Autodesk Inventor part; units mm, degrees
ref_plane "YZ Plane" through (0, 0, 0) normal (1, 0, 0) x (0, 1, 0)
ref_plane "XZ Plane" through (0, 0, 0) normal (0, 1, 0) x (-1, 0, 0)
ref_plane "XY Plane" through (0, 0, 0) normal (0, 0, 1) x (1, 0, 0)
sketch "スケッチ1" plane through (0, 0, 0) normal (1, 0, 0) x (0, 1, 0)
  line L0 (-41, 550) -> (10, 550)
  line L1 (10, 550) -> (10, -10)
  line L2 (10, -10) -> (-41, -10)
  line L3 (-41, -10) -> (-41, 550)
  line L4 (-41, 550) -> (10, -10) construction
  line L5 (10, 550) -> (-41, -10) construction
  point P0 (0, 0)
  dimension "d0" = 51
  dimension "d1" = 560
  dimension "d42" = 10
  dimension "d43" = 10
extrude "プレート1" add sketch "スケッチ1" along normal mid plane 1
sketch "スケッチ3" plane through (0.5, 0, 0) normal (1, 0, 0) x (0, 0, -1)
  circle A0 centre (0, 0) radius 6
  line L0 (10, 10) -> (10, -41)
  line L1 (-550, 10) -> (10, 10)
  point P0 (0, 0)
  point P1 (0, 6)
  point P2 (-6, 0)
  point P3 (0, -6)
  point P4 (6, 0)
  dimension "d13" = 12
  dimension "d14" = 10
  dimension "d15" = 10
  dimension "d18" = 360
  dimension "d44" = 0
hole "穴2" at (0.5, 6, 0) at (0.5, 0, 6) at (0.5, -6, 0) at (0.5, 0, -6) direction (-1, 0, 0) diameter 3.2 end through all
sketch "スケッチ4" plane through (0.5, 0, 0) normal (1, 0, 0) x (0, 0, -1)
  circle A0 centre (0, 0) radius 3.05
  point P0 (0, 0)
  dimension "d27" = 6.1
extrude "押し出し1" cut sketch "スケッチ4" against normal blind 10
sketch "スケッチ5" plane through (0.5, 0, 0) normal (1, 0, 0) x (0, 0, -1)
  line L0 (10, -41) -> (-33.5, -41)
  line L1 (-33.5, -41) -> (-33.5, -10)
  line L2 (-33.5, -10) -> (10, -10)
  line L3 (10, -10) -> (10, -41)
  line L4 (-550, 10) -> (-53.5, 10)
  line L5 (-53.5, 10) -> (-53.5, -12)
  line L6 (-53.5, -12) -> (-550, -12)
  line L7 (-550, -12) -> (-550, 10)
  line L8 (10, -41) -> (-550, -41)
  circle A0 centre (0, 0) radius 3.05
  circle A1 centre (0, 0) radius 3.05
  line L9 (0, 3.05) -> (10, 3.05)
  line L10 (0, -3.05) -> (10, -3.05)
  line L11 (10, 10) -> (10, -41)
  circle A2 centre (0, 0) radius 10
  circle A3 centre (0, 6) radius 1.6
  circle A4 centre (0, -6) radius 1.6
  line L12 (-550, 10) -> (10, 10)
  line L13 (2.95, 10) -> (2.95, -10)
  point P0 (0, 0)
  point P1 (2.95, -3.05)
  point P2 (2.95, 3.05)
  point P3 (2.95, 0.7746)
  point P4 (2.95, -0.7746)
  point P5 (9.5235, -3.05)
  point P6 (0, -10)
  point P7 (0, 10)
  point P8 (9.5235, 3.05)
  point P9 (10, 0)
  point P10 (2.95, -9.555)
  point P11 (2.95, 9.555)
  dimension "d35" = 29
  dimension "d36" = 20
  dimension "d40" = 33.5
  dimension "d41" = 10
  dimension "d45" = 2.95
extrude "押し出し2" cut sketch "スケッチ5" against normal blind 10 contours L0 L1 L2 L3 | L2 L13 A2 L10 L11 | L2 A2 L13 | L10 A2 L11 | L13 L10 A2 | L10 L13 A0 L9 A2 | A2 L9 L11 | L12 L13 A2 | L10 A0 L13 | L9 A2 L13 L12 L11 | L9 L13 A2 | L13 A0 L9 picked at (5.1412, -2.2915)
fillet "コーナーR4" radius 1 4 edges at (0, -3.05, -2.95) (0, 3.05, -2.95) (0, 9.555, -2.95) (0, -9.555, -2.95)
sketch "スケッチ6" plane through (0.5, 0, 0) normal (1, 0, 0) x (0, 0, -1)
  line L0 (-33.5, -41) -> (-550, -41)
  line L1 (-33.5, -41) -> (-33.5, -10)
  line L2 (-33.5, -25) -> (-124.2405, -41)
  point P0 (0, 0)
  point P1 (-545, -41)
  point P2 (-33.5, -15)
  dimension "d51" = 10
  dimension "d52" = 16
extrude "押し出し3" cut sketch "スケッチ6" against normal blind 10
fillet "コーナーR5" radius 5 2 edges at (0, -25, 33.5) (0, -41, 124.2405)
fillet "コーナーR6" radius 5 2 edges at (0, -10, 33.5) (0, 10, 550)
equation "\"d25\" = Thickness"
equation "\"d2\" = Thickness"
equation "\"BendRadius\" = Thickness"
equation "\"BendReliefWidth\" = Thickness"
equation "\"BendReliefDepth\" = 0.5 * Thickness"
equation "\"CornerReliefSize\" = 4 * Thickness"
equation "\"MinimumRemnant\" = 2 * Thickness"
equation "\"TransitionRadius\" = BendRadius"
equation "\"JacobiRadiusSize\" = BendRadius"
equation "\"GapSize\" = Thickness"
properties part number "s_carbon_plate5" material "CFRP"
Source: CAD feature listing. Evaluate the final solid. Frame: model axes, mm. Coordinates: 2 decimals unless noted, no trailing zeros. Write each loop counter-clockwise with the first axis right and the second up, starting at its lowest first coordinate (ties: lowest second). Pieces come first, ordered by that corner, then holes. Notation, with made-up numbers: (77.25, -21.75) - (98.25, -21.75) arc R9 cw to (98.25, -17.75) - close; hole circle Ø4 at (13.5, 83.5). An arc over 180 degrees is marked (long way). Answer as a JSON object with one key per item and string values.
Q1. Section query B-B, the plane y = -31.5. Output: boundary loops of the cut face in (x, z).
Ans:
{"outline": "(-0.5, 70.36) - (0.5, 70.36) - (0.5, 550) - (-0.5, 550) - close"}
Q2. First-contact query: pin 1 Ø0.5 at (x, z) = (0, -1.5) entering from +Y. Flat tip, straight axial feed; report the tip coordinate or a pass-through.
Ans:
{"pin 1": "stops at y = 9.92"}
Q3. Section query A-A, the plane x = -0.05. Output: boundary loops of the cut face in (y, z).
Ans:
{"outline": "(-41, 124.68) arc R5 ccw to (-40.92, 123.81) - (-25.73, 37.63) arc R5 ccw to (-20.8, 33.5) - (-15, 33.5) arc R5 cw to (-10, 28.5) - (-10, 0) arc R10 ccw to (-9.76, -2.17) arc R1 ccw to (-8.79, -2.95) - (-4.05, -2.95) arc R1 ccw to (-3.05, -1.95) - (-3.05, 0) arc R3.05 cw to (3.05, 0) - (3.05, -1.95) arc R1 ccw to (4.05, -2.95) - (8.79, -2.95) arc R1 ccw to (9.76, -2.17) arc R10 ccw to (10, 0) - (10, 545) arc R5 ccw to (5, 550) - (-41, 550) - close; hole circle Ø3.2 at (-6, 0); hole circle Ø3.2 at (0, 6); hole circle Ø3.2 at (6, 0)"}
Q4. Material intervals for line 1 (Y direction, x = 0, z = 0); line 2 (Z direction, x = -0.1, y = 6); line 3 (Z direction, x = -0.15, y = -6), sorted ascending. Write a range as [from, to].
Ans:
{"line 1": "y = [-10, -7.6], [-4.4, -3.05], [3.05, 4.4], [7.6, 10]", "line 2": "z = [-2.95, -1.6], [1.6, 549.9]", "line 3": "z = [-2.95, -1.6], [1.6, 550]"}
Q5. Section query C-C, the plane z = 50.5. Output: boundary loops of the cut face in (x, y).
Ans:
{"outline": "(-0.5, -28) - (0.5, -28) - (0.5, 10) - (-0.5, 10) - close"}
